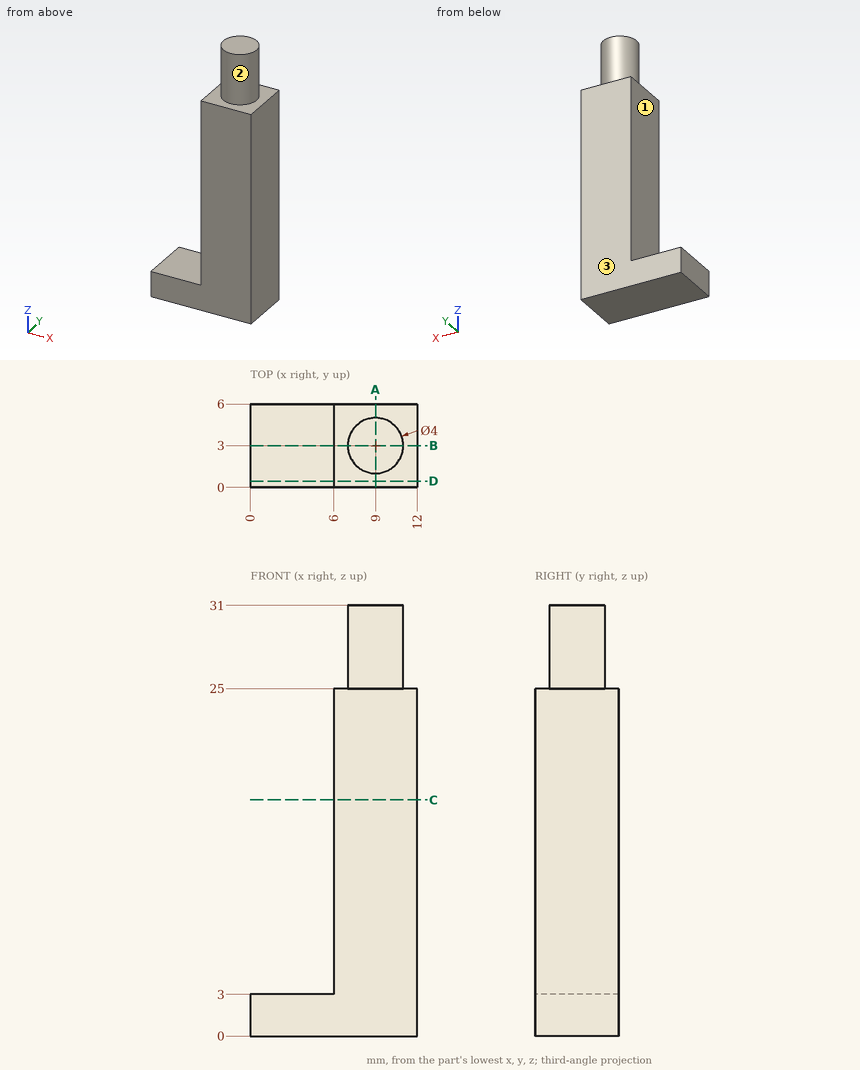
Input: dimensioned drawing with shaded views. Units: mm. Origin: part minimum x, y, z. A direction names the side the tool comes from. Coordinates: 2 decimals unless noted, no trailing zeros. Write each loop counter-clockwise with the first axis right and the second up, starting at its lowest first coordinate (ties: lowest second). Pieces come first, ordered by that corner, then holes. Notation, with made-up numbers: M 66,70.5 L 87,70.5 A22 cw 87,92.5 Z; hole C 64.25,18 d4. An arc over 180 degrees is marked long. Answer as a JSON object with one key per item and string values. Group by question number.
(1) Section C-C on z = 17. Output: boundary loops of the cut face in (x, y).
(2) Section D-D on y = 0.45. Output: boundary loops of the cut face in (x, z).
(3) Ray query, line 1 along X through (y, z) = (0.9, 22.5); line 2 along Z through (x, y) = (3.75, 5.75); line 3 along Z through (x, y) = (11.5, 2.95). Return the intervals inside material, ascending. Write a range as [from, to].
(4) Set-up query: the marked faces 1, 2 and 3. Return all of +Z, -Z, +X, -X, +Y, -Y with unobstructed straight access to the full face (end or side cutting, diameter ignored); none if empty.
(5) Section B-B on y = 3. Output: boundary loops of the cut face in (x, z), plus the area to 3 significant figures.
(6) Contact query for a flat-ended pin moving along its axis: P1, Ø2, axis at y = 4.5, z = 14, coming from the -X side. Output: stop coordinate, or through.
(7) Section A-A on x = 9. Output: boundary loops of the cut face in (y, z).
Result set:
{
 "1": {"outline": "M 6,0 L 12,0 L 12,6 L 6,6 Z"},
 "2": {"outline": "M 0,0 L 12,0 L 12,25 L 6,25 L 6,3 L 0,3 Z"},
 "3": {"line 1": "x = [6, 12]", "line 2": "z = [0, 3]", "line 3": "z = [0, 25]"},
 "4": {"face 1": "+Z, -X, +Y, -Y", "face 2": "+Z", "face 3": "+Z, -Z, +X, -X, +Y"},
 "5": {"outline": "M 0,0 L 12,0 L 12,25 L 11,25 L 11,31 L 7,31 L 7,25 L 6,25 L 6,3 L 0,3 Z", "area": "192 mm2"},
 "6": {"P1": "stops at x = 6"},
 "7": {"outline": "M 0,0 L 6,0 L 6,25 L 5,25 L 5,31 L 1,31 L 1,25 L 0,25 Z"}
}
